Input: part model. Units: mm. Frame: model coordinates. A direction names the side the tool comes from. Round coordinates to 2 decimals unless told otherwise and drop trailing zeros. Loops run counter-clockwise (first coordinate to the right, second up) from the corner with the lowest first, then second, coordinate; pieces in that order, holes last. Notation, with made-up numbers: (29.25, 88) -> (49.25, 88) arc R23 ccw to (49.25, 114) -> close; hole circle Ø2 at (84.25, 14.5). An arc over 180 degrees is marked (long way). Answer in a Markdown table with one row per item. Add a question column.
Q1. Mould query, pull axis Z, two halves, no side actions, for faces 6 (the face through (69.113, 73, -49)), 7 (the face through (86, 71, -100)), 8 (the face through (74, 145, -9)). Classes: pulls with the +Z half, pulls with the -Z half, needs draft (parallel to the pull), parting line crosses it, or undercut.
Q2. Ray query, L1, parallel to X at y = 32.5, z = -65.5; L2, parallel to X at y = 83, z = -50; L3, parallel to X at y = 120, z = -83. Return the intervals inside material, ascending. Write a range as from..to.
Q3. Section D-D, the plane z = -44. Output: boundary loops of the cut face in (x, y), and give its area (3 significant figures).
Q4. Section B-B, the plane y = 59. Output: boundary loops of the cut face in (x, z), and give its area (3 significant figures).
Q5. Section A-A, the plane x = 64. Output: boundary loops of the cut face in (y, z), and give its area (3 significant figures).
Q6. Section C-C, the plane z = -70. Output: boundary loops of the cut face in (x, y), and give its area (4 significant figures).
Q7. Pin query (flat end, axial travel): pin 1 (8 mm diameter, centred on x = 72, z = -71.5, fed in from -Y); pin 2 (18 mm diameter, centred on x = 86.61, z = -50, fed in from -Y) (1 decimal). Return the tip coordinate at first contact, or that it passes through.
Q8. Reachability of faces 1 (the face through (75, 115, -51)), 2 (the face through (175, 71, -49)), 3 (the face through (86, 71, 0)), 4 (the face through (75, 30, -49)), 5 (the face through (10, 74, -49)) from +Z, -Z, +X, -X, +Y, -Y: full face, straight path, thin tool, end or side. Return the list, or none.
```python
from build123d import *

# Parameters (mm, degrees)
SKETCH1_W           = 175
SKETCH1_H           = 100
BOSS_EXTRUDE1_DEPTH = 145
SKETCH2_R           = 11.25
SKETCH2_W           = 59.113281673
SKETCH2_H           = 80
SKETCH2_W_2         = 60.886718327
CUT_EXTRUDE1_DEPTH  = 145
SKETCH4_W           = 35
SKETCH4_H           = 80
CUT_EXTRUDE2_DEPTH  = 30
SKETCH5_W           = 35
SKETCH5_H           = 80
CUT_EXTRUDE3_DEPTH  = 30


with BuildPart() as part:
    # Sketch1 → Boss-Extrude1 (new body)
    with BuildSketch(Plane(origin=(0, 0, 0), x_dir=(1, 0, 0), z_dir=(0, 1, 0))):
        with Locations((87.5, 50)):
            Rectangle(SKETCH1_W, SKETCH1_H)
    extrude(amount=BOSS_EXTRUDE1_DEPTH)

    # Sketch2 → Cut-Extrude1 (cut)
    with BuildSketch(Plane(origin=(0, 145, 0), x_dir=(1, 0, 0), z_dir=(0, 1, 0))):
        with Locations((86.613281673, 50)):
            Circle(SKETCH2_R)
        with Locations((39.556640837, 50)):
            Rectangle(SKETCH2_W, SKETCH2_H)
        with Locations((134.556640837, 50)):
            Rectangle(SKETCH2_W_2, SKETCH2_H)
    extrude(amount=-CUT_EXTRUDE1_DEPTH, mode=Mode.SUBTRACT)

    # Sketch4 → Cut-Extrude2 (cut)
    with BuildSketch(Plane(origin=(0, 145, 0), x_dir=(1, 0, 0), z_dir=(0, 1, 0))):
        with Locations((86.613281673, 50)):
            Rectangle(SKETCH4_W, SKETCH4_H)
    extrude(amount=-CUT_EXTRUDE2_DEPTH, mode=Mode.SUBTRACT)

    # Sketch5 → Cut-Extrude3 (cut)
    with BuildSketch(Plane.XZ):
        with Locations((86.613281673, -50)):
            Rectangle(SKETCH5_W, SKETCH5_H)
    extrude(amount=-CUT_EXTRUDE3_DEPTH, mode=Mode.SUBTRACT)


solid = part.part
```
Answer block:
| question | item | result |
|---|---|---|
| 1 | face 6 | undercut |
| 1 | face 7 | pulls with the -Z half |
| 1 | face 8 | needs draft |
| 2 | L1 | 0..10, 69.11..104.11, 165..175 |
| 2 | L2 | 0..10, 69.11..75.36, 97.86..104.11, 165..175 |
| 2 | L3 | 0..10, 165..175 |
| 3 | outline | (0, 0) -> (10, 0) -> (10, 145) -> (0, 145) -> close; (69.11, 30) -> (77.1, 30) -> (77.1, 115) -> (69.11, 115) -> close; (96.13, 30) -> (104.11, 30) -> (104.11, 115) -> (96.13, 115) -> close; (165, 0) -> (175, 0) -> (175, 145) -> (165, 145) -> close |
| 3 | area | 4,260 mm^2 |
| 4 | outline | (0, -100) -> (175, -100) -> (175, 0) -> (0, 0) -> close; hole (10, -90) -> (69.11, -90) -> (69.11, -10) -> (10, -10) -> close; hole circle Ø22.5 at (86.61, -50); hole (104.11, -90) -> (165, -90) -> (165, -10) -> (104.11, -10) -> close |
| 4 | area | 7,500 mm^2 |
| 5 | outline | (0, -100) -> (145, -100) -> (145, -90) -> (0, -90) -> close; (0, -10) -> (145, -10) -> (145, 0) -> (0, 0) -> close |
| 5 | area | 2,900 mm^2 |
| 6 | outline | (0, 0) -> (10, 0) -> (10, 145) -> (0, 145) -> close; (69.11, 30) -> (104.11, 30) -> (104.11, 115) -> (69.11, 115) -> close; (165, 0) -> (175, 0) -> (175, 145) -> (165, 145) -> close |
| 6 | area | 5,875 mm^2 |
| 7 | pin 1 | y = 30 |
| 7 | pin 2 | through |
| 8 | face 1 | +Y |
| 8 | face 2 | +Z, -Z, +X, +Y, -Y |
| 8 | face 3 | +Z, +X, -X, +Y, -Y |
| 8 | face 4 | -Y |
| 8 | face 5 | +Y, -Y |
